Read the model definition and answer for the solid it produces. Units are mm, in the model's axes. A direction names the side the tool comes from. Give positions to 0.01 mm unless a question says otherwise; leave off trailing zeros. Write each loop counter-clockwise with the first axis right and the second up, starting at its lowest first coordinate (ties: lowest second). Pieces come first, ordered by that corner, then holes. Notation, with made-up numbers: (52.25, 53.5) -> (94.25, 53.5) arc R22 cw to (94.25, 73.5) -> close; hole circle Ø4 at (78, 39). An arc over 180 degrees is marked (long way). Write item = value, one per line.
from build123d import *

# Parameters (mm, degrees)
SKETCH1_W           = 48.26
SKETCH1_H           = 17.018
BOSS_EXTRUDE1_DEPTH = 16.9164
SKETCH3_W           = 38.503555909
SKETCH3_H           = 15.229875851
CUT_EXTRUDE1_DEPTH  = 7.62
SKETCH4_W           = 6.096
SKETCH4_H           = 14.944038535
CUT_EXTRUDE2_DEPTH  = 15.24
SKETCH5_W           = 15.494422394
SKETCH5_H           = 11.468029568
SKETCH5_W_2         = 16.429120729
SKETCH5_H_2         = 11.755629056
BOSS_EXTRUDE2_DEPTH = 5.08


with BuildPart() as part:
    # Sketch1 → Boss-Extrude1 (new body)
    with BuildSketch(Plane(origin=(0, 0, 0), x_dir=(1, 0, 0), z_dir=(0, 1, 0))):
        with Locations((24.13, 8.509)):
            Rectangle(SKETCH1_W, SKETCH1_H)
    extrude(amount=BOSS_EXTRUDE1_DEPTH)

    # Sketch3 → Cut-Extrude1 (cut)
    with BuildSketch(Plane(origin=(0, 0, -17.018), x_dir=(-1, 0, 0), z_dir=(0, 0, -1))):
        with Locations((-24.292361965, 9.301462074)):
            Rectangle(SKETCH3_W, SKETCH3_H)
    extrude(amount=-CUT_EXTRUDE1_DEPTH, mode=Mode.SUBTRACT)

    # Sketch4 → Cut-Extrude2 (cut)
    with BuildSketch(Plane(origin=(0, 1.686524149, 0), x_dir=(1, 0, 0), z_dir=(0, 1, 0))):
        with Locations((17.651266973, 9.545980733)):
            Rectangle(SKETCH4_W, SKETCH4_H)
        with Locations((30.19779462, 9.545980733)):
            Rectangle(SKETCH4_W, SKETCH4_H)
    extrude(amount=CUT_EXTRUDE2_DEPTH, mode=Mode.SUBTRACT)

    # Sketch5 → Boss-Extrude2 (add)
    with BuildSketch(Plane(origin=(0, 16.9164, 0), x_dir=(1, 0, 0), z_dir=(0, 1, 0))):
        with Locations((-3.20992629, 8.562924904)):
            Rectangle(SKETCH5_W, SKETCH5_H)
        with Locations((52.224874945, 8.41912516)):
            Rectangle(SKETCH5_W_2, SKETCH5_H_2)
    extrude(amount=BOSS_EXTRUDE2_DEPTH)


solid = part.part
(1) Consider L1, parallel to X at y = 1.75, z = -4; L2, parallel to X at y = 5.5, z = -15; L3, parallel to Y at x = 16.5, z = -9.25. Determine where each line is inside the solid, lowest interval first.
Checks:
L1 = 0 to 14.6, 20.7 to 27.15, 33.25 to 48.26
L2 = 0 to 5.04, 43.54 to 48.26
L3 = 0 to 1.69
(2) The part is cut by section A-A on y = 19.25. Determine the outline of the cut face in (x, z), plus the area to 3 significant figures.
Checks:
outline = (-10.96, -14.3) -> (4.54, -14.3) -> (4.54, -2.83) -> (-10.96, -2.83) -> close; (44.01, -14.3) -> (60.44, -14.3) -> (60.44, -2.54) -> (44.01, -2.54) -> close
area = 371 mm²
(3) Given P1, Ø3.5, axis at y = 9.5, z = -7.5, coming from the -X side; P2, Ø6, axis at y = 12.5, z = -11.5, coming from the +X side; P3, Ø5, axis at x = 39.5, y = 12.5, coming from the -Z side; P4, Ø2, axis at x = 2.5, y = 11.5, coming from the +Z side, each flat-ended and moving along its own axis, determine where each tip first touches the part or whether it passes through.
Checks:
P1 = 0
P2 = 48.26
P3 = -9.4
P4 = 0
(4) The part is cut by section C-C on z = -5. Determine the outline of the cut face in (x, y), plus the area to 3 significant figures.
Checks:
outline = (-10.96, 16.92) -> (0, 16.92) -> (0, 0) -> (48.26, 0) -> (48.26, 16.92) -> (60.44, 16.92) -> (60.44, 22) -> (44.01, 22) -> (44.01, 16.92) -> (33.25, 16.92) -> (33.25, 1.69) -> (27.15, 1.69) -> (27.15, 16.92) -> (20.7, 16.92) -> (20.7, 1.69) -> (14.6, 1.69) -> (14.6, 16.92) -> (4.54, 16.92) -> (4.54, 22) -> (-10.96, 22) -> close
area = 793 mm²
(5) A tool of negligible diameter and unlimited length cuts with its end or side. For faces 5 (the flat face through (52, 19, -2.541)), 6 (the flat face through (14.603, 9, -6)), 7 (the flat face through (-6, 16.916, -9)), 8 (the flat face through (4.537, 19, -8)), from which of +Z, -Z, +X, -X, +Y, -Y can it reach the whole face along a straight path? Write none if from no direction.
Checks:
face_5 = +Z, +X, -X, +Y
face_6 = -Z, +Y
face_7 = +Z, -Z, -X, -Y
face_8 = +Z, -Z, +Y
(6) The part is cut by section D-D on y = 6.5. Determine the outline of the cut face in (x, z), plus the area to 3 significant figures.
Checks:
outline = (0, -17.02) -> (5.04, -17.02) -> (5.04, -9.4) -> (14.6, -9.4) -> (14.6, -2.07) -> (20.7, -2.07) -> (20.7, -9.4) -> (27.15, -9.4) -> (27.15, -2.07) -> (33.25, -2.07) -> (33.25, -9.4) -> (43.54, -9.4) -> (43.54, -17.02) -> (48.26, -17.02) -> (48.26, 0) -> (0, 0) -> close
area = 439 mm²
(7) The part is cut by section B-B on x = 47. Determine the outline of the cut face in (y, z), plus the area to 3 significant figures.
Checks:
outline = (0, -17.02) -> (16.92, -17.02) -> (16.92, -14.3) -> (22, -14.3) -> (22, -2.54) -> (16.92, -2.54) -> (16.92, 0) -> (0, 0) -> close
area = 348 mm²
(8) For a pull along X with two mould halves and no side action, classify faces 1 (the flat face through (48.26, 8, -8)), 2 (the flat face through (-10.957, 19, -8)), 3 (the flat face through (44.01, 19, -8)), 4 (the flat face through (52, 19, -14.297)) as released by +X, released by -X, zero draft, split by the parting line, or undercut.
Checks:
face_1 = released by +X
face_2 = released by -X
face_3 = undercut
face_4 = zero draft
